CAD build for the part. Positions are in the model's coordinates, mm. A direction names the side the tool comes from. Round coordinates to 2 decimals unless told otherwise and drop trailing zeros. Order: outer loops, then holes, each group sorted by start corner. A loop starts at its lowest first (then second) coordinate and runs counter-clockwise, first axis right, second up.
Autodesk Inventor part; units mm, degrees
ref_plane "YZ Plane" through (0, 0, 0) normal (1, 0, 0) x (0, 1, 0)
ref_plane "XZ Plane" through (0, 0, 0) normal (0, 1, 0) x (-1, 0, 0)
ref_plane "XY Plane" through (0, 0, 0) normal (0, 0, 1) x (1, 0, 0)
sketch "Boceto1" plane through (0, 0, 0) normal (0, 0, 1) x (1, 0, 0)
  line L0 (-4.5, 15.5) -> (-4.5, 12.5)
  line L1 (-4.5, 12.5) -> (-9.5, 12.5)
  line L2 (-9.5, 12.5) -> (-9.5, -12.5)
  line L3 (-9.5, -12.5) -> (-4.5, -12.5)
  line L4 (-4.5, -12.5) -> (-4.5, -15.5)
  line L5 (-4.5, -15.5) -> (-1.5, -15.5)
  line L6 (-1.5, 15.5) -> (-4.5, 15.5)
  line L7 (9.5, 12.5) -> (9.5, -12.5)
  line L8 (9.5, -12.5) -> (4.5, -12.5)
  line L9 (4.5, -12.5) -> (4.5, -15.5)
  line L10 (4.5, -15.5) -> (-4.5, -15.5)
  line L11 (-4.5, 15.5) -> (4.5, 15.5)
  line L12 (4.5, 15.5) -> (4.5, 12.5)
  line L13 (4.5, 12.5) -> (9.5, 12.5)
extrude "Extrusión1" add sketch "Boceto1" along normal blind 3
properties part number "Wall_Base2" material "MDF Tablero de fibras de densidad media"
1. Cut at B-B, the plane x = -6.25. Write the cut outline in (y, z), and give its area (3 significant figures).
2. Cut at A-A, the plane z = 0.35. Write the cut outline in (x, y).
3. Pin check, flat tips, straight feed: P1, Ø1.5, axis at y = 13.5, z = 2, coming from the +X side; P2, Ø0.9, axis at x = -6.5, z = 1, coming from the -Y side; P3, Ø0.9, axis at x = -6.5, z = 2, coming from the +Y side. Stop position of each tip, or through.
4. Drill centre lines: line 1 (Y direction, x = -8, z = 1.55); line 2 (X direction, y = 14.5, z = 2.7). Where is each one in solid material? Low to high.
5. Tool access for faces 1 (the face through (4.5, 14, 1)), 2 (the face through (-4.5, -14, 1)), 3 (the face through (7, -12.5, 1)), 4 (the face through (-4.5, 14, 1)): list every direction of +Z, -Z, +X, -X, +Y, -Y with a clear straight run to the whole face (end or side of a thin tool).
Outcome:
1. outline: (-12.5, 0) - (12.5, 0) - (12.5, 3) - (-12.5, 3) - close
1. area: 75.0 mm2
2. outline: (-9.5, -12.5) - (-4.5, -12.5) - (-4.5, -15.5) - (4.5, -15.5) - (4.5, -12.5) - (9.5, -12.5) - (9.5, 12.5) - (4.5, 12.5) - (4.5, 15.5) - (-4.5, 15.5) - (-4.5, 12.5) - (-9.5, 12.5) - close
3. P1: stops at x = 4.5
3. P2: stops at y = -12.5
3. P3: stops at y = 12.5
4. line 1: y = -12.5 to 12.5
4. line 2: x = -4.5 to 4.5
5. face 1: +Z, -Z, +X, +Y
5. face 2: +Z, -Z, -X, -Y
5. face 3: +Z, -Z, +X, -Y
5. face 4: +Z, -Z, -X, +Y
